Verification items for the finished model (mm, model axes). A direction names the side the tool comes from. Coordinates: 2 decimals unless noted, no trailing zeros. Loops run counter-clockwise (first coordinate to the right, second up) from the corner with the lowest first, then second, coordinate; pieces in that order, holes last.
Q1. Sectioned sample at C-C (x = -16). Enter the section's corners in (y, z), then the cut area to 3 significant figures.
Q2. Sectioned sample at D-D (y = 6.5). Enter the section's corners in (x, z), then the cut area to 3 significant figures.
Q3. Sectioned sample at B-B (z = 1.25). Enter the section's corners in (x, y), then the cut area to 3 significant figures.
Q4. Material ranges on probe 1 along X at (y, z) = (21, 0.7); probe 2 along X at (y, z) = (-11.5, 2.2); probe 3 along X at (y, z) = (12, 0.65), recorded low to high.
Q5. Go/stop test with flat-tipped pins: P1, Ø3.5, axis at x = -24.61, y = 22.67, coming from the -Z side; P2, Ø1, axis at x = 1.5, z = 1.5, coming from the -Y side; P3, Ø1.2, axis at y = -14.5, z = 1, coming from the -X side. Record where each tip stops, or that it passes through.
Q6. Mould release check, pull along X, two halves, no side actions. Record for faces 1 (the face through (15.394, -3, 1)), 2 (the face through (1, 33.075, 1)), 3 (the face through (6.394, -16, 1)): +X half, -X half, draft (parallel to the pull), parting line (faces both ways), or undercut.
Q7. Access from +Z, -Z, +X, -X, +Y, -Y to the whole of each face (thin tool, end or side, straight path). Record for faces 4 (the face through (-2.465, -7.928, 1.183)), 5 (the face through (-12.606, -3, 1)), 6 (the face through (2, 12, 0)).
Q8. Sectioned sample at A-A (y = -16). Enter the section's corners in (x, z).
```python
from build123d import *

# Parameters (mm, degrees)
SKETCH1_R           = 2.15
BOSS_EXTRUDE1_DEPTH = 2.4
SKETCH2_W           = 10
SKETCH2_H           = 30
CUT_EXTRUDE1_DEPTH  = 3.4
FILLET1_R           = 4


with BuildPart() as part:
    # Sketch1 → Boss-Extrude1 (new body)
    with BuildSketch(Plane.XY):
        Polygon((-21.105584483, 33.074652619), (23.894415517, 33.074652619), (33.894415517, 23.074652619), (33.894415517, 16.074652619), (15.394415517, 16.074652619), (15.394415517, -21.725347381), (-12.605584483, -21.725347381), (-12.605584483, 16.074652619), (-31.105584483, 16.074652619), (-31.105584483, 23.074652619), align=None)
        with Locations((-24.605584483, 22.674652619)):
            Circle(SKETCH1_R, mode=Mode.SUBTRACT)
        with Locations((27.394415517, 22.674652619)):
            Circle(SKETCH1_R, mode=Mode.SUBTRACT)
    extrude(amount=BOSS_EXTRUDE1_DEPTH)

    # Sketch2 → Cut-Extrude1 (cut, through all)
    with BuildSketch(Plane.XY.offset(2.4)):
        with Locations((1.394415517, -21.725347381)):
            Rectangle(SKETCH2_W, SKETCH2_H)
    extrude(amount=-CUT_EXTRUDE1_DEPTH, mode=Mode.SUBTRACT)

    # Fillet1
    fillet1_edges = [part.edges().sort_by_distance(p)[0] for p in [
        (6.394415517, -6.725347381, 1.2),
        (-3.605584483, -6.725347381, 1.2),
    ]]
    fillet(fillet1_edges, radius=FILLET1_R)


solid = part.part
```
Geometry check:
1. outline: (16.07, 0) - (33.07, 0) - (33.07, 2.4) - (16.07, 2.4) - close
1. area: 40.8 mm2
2. outline: (-12.61, 0) - (15.39, 0) - (15.39, 2.4) - (-12.61, 2.4) - close
2. area: 67.2 mm2
3. outline: (-31.11, 16.07) - (-12.61, 16.07) - (-12.61, -21.73) - (-3.61, -21.73) - (-3.61, -10.73) arc R4 cw to (0.39, -6.73) - (2.39, -6.73) arc R4 cw to (6.39, -10.73) - (6.39, -21.73) - (15.39, -21.73) - (15.39, 16.07) - (33.89, 16.07) - (33.89, 23.07) - (23.89, 33.07) - (-21.11, 33.07) - (-31.11, 23.07) - close; hole circle Ø4.3 at (-24.61, 22.67); hole circle Ø4.3 at (27.39, 22.67)
3. area: 1,890 mm2
4. probe 1: x = -31.11 to -25.95, -23.26 to 26.05, 28.74 to 33.89
4. probe 2: x = -12.61 to -3.61, 6.39 to 15.39
4. probe 3: x = -12.61 to 15.39
5. P1: passes through
5. P2: stops at y = -6.73
5. P3: stops at x = -12.61
6. face 1: +X half
6. face 2: draft
6. face 3: undercut
7. face 4: +Z, -Z, -Y
7. face 5: +Z, -Z, -X, -Y
7. face 6: -Z, +X, -X, +Y, -Y
8. outline: (-12.61, 0) - (-3.61, 0) - (-3.61, 2.4) - (-12.61, 2.4) - close; (6.39, 0) - (15.39, 0) - (15.39, 2.4) - (6.39, 2.4) - close
